Work out the finished part from the listing and answer in its coordinate system (mm). Face numbers are marked on the shaded views. Coordinates: 2 decimals unless noted, no trailing zeros. Write each loop counter-clockwise with the first axis right and the second up, starting at its lowest first coordinate (ties: lowest second). Pieces come first, ordered by that corner, then holes. Notation, with made-up numbers: M 76,-23 L 105,-23 A15 cw 105,-8 Z; hole C 35.25,65.25 d8. An arc over 180 degrees is marked long. Answer as CSV lines item,"result". Start each with the question number.
(1) Find the intervals of material crossed by L1, parallel to X at y = -17, z = -66.5; L2, parallel to Y at x = 60, z = -50; L3, parallel to Z at x = 43.25, y = -31.5, in increasing order. Write a range as [from, to].
(2) A cutting plane is placed at C-C on y = -31.5. Count the separate pieces of the cut face and the enclosed holes in it, then the cut area to 3 significant figures.
(3) The mould has two halves that part along X. Classify the marked faces 1, 2 and 3: released by +X, released by -X, zero draft, split by the parting line, or undercut.
(4) A cutting plane is placed at B-B on z = -82. Give the vertices of the cut face in (x, y), then the cut area to 3 significant figures.
(5) Flat-ended cylindrical pins translate along their axes: P1, Ø1, axis at y = -5.5, z = -68, coming from the -X side; P2, Ø7, axis at x = 48.4, z = -45.33, coming from the -Y side; P3, Ø10, axis at y = -23, z = -66, coming from the -X side; P4, Ø7, axis at y = -31.5, z = -64.33, coming from the -X side. Find the tip coordinate at first contact, or state that the pin passes through.
(6) A cutting plane is placed at D-D on z = -51. Give the vertices of the cut face in (x, y), then the cut area to 3 significant figures.
(7) A cutting plane is placed at A-A on y = -24. Give the vertices of the cut face in (x, z).
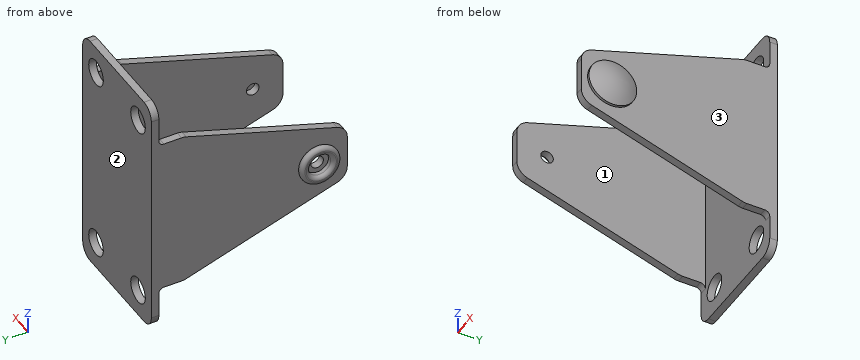
from build123d import *

# Parameters (mm, degrees)
SKETCH_1_W          = 24.5
SKETCH_1_H          = 49
EXTRUDE_1_DEPTH     = 1.5
EXTRUDE_2_DEPTH     = 1.5
EXTRUDE_3_DEPTH     = 1.5
SKETCH_5_R          = 2.6
CUT_EXTRUDE_1_DEPTH = 119.55472929
FILLET_1_R          = 2.6
SKETCH_6_R          = 1.25
CUT_EXTRUDE_2_DEPTH = 100.482631552
FILLET_2_R          = 3
FILLET_3_R          = 1


with BuildPart() as part:
    # 草图1 → 凸台-拉伸1 (new body)
    with BuildSketch(Plane(origin=(0, 0, 0), x_dir=(1, 0, 0), z_dir=(0, 1, 0))):
        with Locations((55.896385498, 64.327326767)):
            Rectangle(SKETCH_1_W, SKETCH_1_H)
    extrude(amount=EXTRUDE_1_DEPTH)

    # 草图2 → 凸台-拉伸2 (add)
    with BuildSketch(Plane(origin=(68.146385498, 0, 0), x_dir=(0, 0, -1), z_dir=(1, 0, 0))):
        Polygon((69.827326767, -37.5), (58.827326767, -37.5), (48.327326767, -5), (48.327326767, 1.5), (64.327326767, 1.5), (80.327326767, 1.5), (80.327326767, -5), align=None)
    extrude(amount=-EXTRUDE_2_DEPTH)

    # 草图4 → 凸台-拉伸3 (add)
    with BuildSketch(Plane.ZY.offset(-43.646385498)):
        Polygon((-48.327326767, -5), (-48.327326767, 0), (-80.327326767, 0), (-80.327326767, -5), (-69.827326767, -37.5), (-58.827326767, -37.5), align=None)
    extrude(amount=-EXTRUDE_3_DEPTH)

    # 草图5 → 切除-拉伸1 (cut, through all)
    with BuildSketch(Plane(origin=(0, 1.5, 0), x_dir=(1, 0, 0), z_dir=(0, 1, 0))):
        with Locations(Location((48.396385498, 83.327326767, 0), (0, 0, 270))):
            Circle(SKETCH_5_R)
        with Locations(Location((63.396385498, 83.327326767, 0), (0, 0, 270))):
            Circle(SKETCH_5_R)
        with Locations(Location((63.396385498, 45.327326767, 0), (0, 0, 90))):
            Circle(SKETCH_5_R)
        with Locations(Location((48.396385498, 45.327326767, 0), (0, 0, 90))):
            Circle(SKETCH_5_R)
    extrude(amount=-CUT_EXTRUDE_1_DEPTH, mode=Mode.SUBTRACT)

    # 圆角1
    fillet_1_edges = [part.edges().sort_by_distance(p)[0] for p in [
        (43.646385498, 0.75, -39.827326767),
        (43.646385498, 0.75, -88.827326767),
        (68.146385498, 0.75, -88.827326767),
        (68.146385498, 0.75, -39.827326767),
    ]]
    fillet(fillet_1_edges, radius=FILLET_1_R)

    # 草图6 → 切除-拉伸2 (cut, through all)
    with BuildSketch(Plane.ZY.offset(-43.646385498)):
        with Locations((-64.327326767, -31.5)):
            Circle(SKETCH_6_R)
    extrude(amount=-CUT_EXTRUDE_2_DEPTH, mode=Mode.SUBTRACT)

    # 圆角2
    fillet_2_edges = [part.edges().sort_by_distance(p)[0] for p in [
        (67.396385498, -5, -80.327326767),
        (67.396385498, -37.5, -69.827326767),
        (67.396385498, -37.5, -58.827326767),
        (67.396385498, -5, -48.327326767),
        (44.396385498, -5, -48.327326767),
        (44.396385498, -37.5, -58.827326767),
        (44.396385498, -37.5, -69.827326767),
        (44.396385498, -5, -80.327326767),
    ]]
    fillet(fillet_2_edges, radius=FILLET_2_R)

    # 圆角3
    fillet_3_edges = [part.edges().sort_by_distance(p)[0] for p in [
        (67.396385498, 0, -48.327326767),
        (67.396385498, 0, -80.327326767),
        (44.396385498, 0, -80.327326767),
        (44.396385498, 0, -48.327326767),
    ]]
    fillet(fillet_3_edges, radius=FILLET_3_R)

    # 草图9 → 旋转1 (revolve)
    with BuildSketch(Plane(origin=(0, 0, -64.327326767), x_dir=(-1, 0, 0), z_dir=(0, 0, 1))):
        with BuildLine():
            Line((-68.146385498, 31.5), (-68.146385498, 26.75))
            Line((-68.146385498, 26.75), (-68.646385498, 26.75))
            ThreePointArc((-68.646385498, 26.75), (-69.762475458, 29.009392644), (-70.146385498, 31.5))
            Line((-70.146385498, 31.5), (-68.146385498, 31.5))
        make_face()
    revolve(axis=Axis((68.146385498, -31.5, -64.327326767), (1, 0, 0)))

    # 草图10 → 旋转2 (revolve)
    with BuildSketch(Plane(origin=(0, 0, -64.327326767), x_dir=(-1, 0, 0), z_dir=(0, 0, 1)), mode=Mode.PRIVATE) as revolve_2_sk:
        with BuildLine():
            Line((-42.146385498, 28.5), (-42.146385498, 28.25))
            ThreePointArc((-42.146385498, 28.25), (-42.896385498, 27.5), (-43.646385498, 28.25))
            Line((-43.646385498, 28.25), (-43.646385498, 29.25))
            Line((-43.646385498, 29.25), (-42.896385498, 29.25))
            ThreePointArc((-42.896385498, 29.25), (-42.366055412, 29.030330086), (-42.146385498, 28.5))
        make_face()
    revolve(revolve_2_sk.sketch.rotate(Axis((68.146385498, -31.5, -64.327326767), (-1, 0, 0)), 90), axis=Axis((68.146385498, -31.5, -64.327326767), (-1, 0, 0)))


solid = part.part
Here are the results:
1,L1,"x = [43.65, 45.15], [66.65, 68.15]"
1,L2,"y = [0, 1.5]"
1,L3,"z = [-68.24, -66.58], [-62.08, -60.42]"
2,separate pieces,"3"
2,enclosed holes,"0"
2,area,"56.1 mm^2"
3,face 1,"undercut"
3,face 2,"zero draft"
3,face 3,"released by +X"
4,outline,"M 43.65,0 L 46.16,0 L 46.16,1.5 L 43.65,1.5 Z; M 50.63,0 L 61.16,0 L 61.16,1.5 L 50.63,1.5 Z; M 65.63,0 L 68.15,0 L 68.15,1.5 L 65.63,1.5 Z"
4,area,"23.3 mm^2"
5,P1,"stops at x = 43.65"
5,P2,"stops at y = 0"
5,P3,"stops at x = 42.27"
5,P4,"stops at x = 42.15"
6,outline,"M 43.65,-13.27 L 45.15,-13.27 L 45.15,0 L 66.65,0 L 66.65,-13.27 L 68.15,-13.27 L 68.15,1.5 L 43.65,1.5 Z"
6,area,"76.6 mm^2"
7,outline,"M 43.65,-74.19 L 45.15,-74.19 L 45.15,-54.47 L 43.65,-54.47 Z; M 66.65,-74.19 L 68.15,-74.19 L 68.15,-54.47 L 66.65,-54.47 Z"
